Here's the drawing with two shaded views (mm, measured from the low corner). I have some questions. A direction names the side the tool comes from. Give positions to 0.01 mm unless a question says otherwise; leave off trailing zeros. Loops run counter-clockwise (first coordinate to the right, second up) from the corner with the lowest first, then second, coordinate; pieces in that order, holes last.
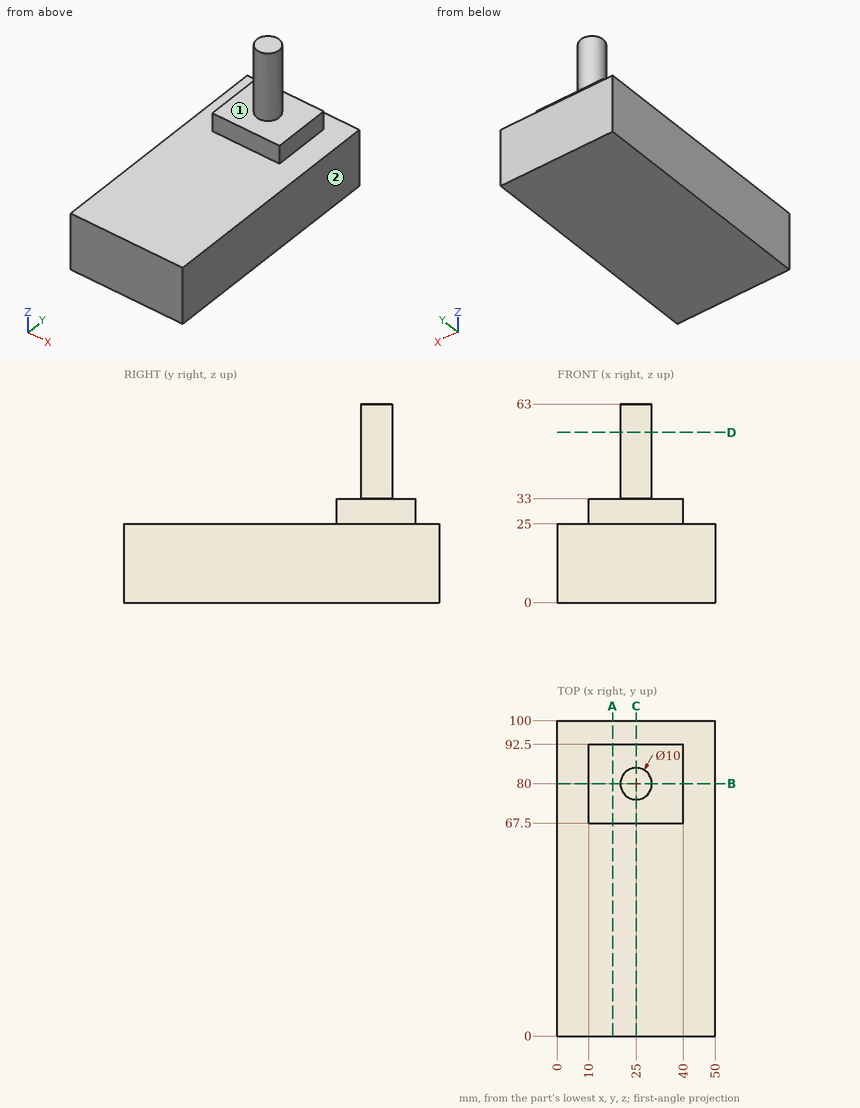
(1) Suppose I cut it at C-C on x = 25. List the corners of the cut face in (y, z) for me.
Returned:
outline: (0, 0) - (100, 0) - (100, 25) - (92.5, 25) - (92.5, 33) - (85, 33) - (85, 63) - (75, 63) - (75, 33) - (67.5, 33) - (67.5, 25) - (0, 25) - close
(2) Which directions (+Z, -Z, +X, -X, +Y, -Y) give clear straight access to the entire face, cutting with the end or side of a thin tool? Please do the marked faces 1 and 2.
Returned:
face 1: +Z
face 2: +Z, -Z, +X, +Y, -Y
(3) Please list where these lines run through material, in increasing order: probe 1 along Z at (x, y) = (18, 58); probe 2 along Y at (x, z) = (19, 29.5); probe 3 along Z at (x, y) = (32, 75.5).
Returned:
probe 1: z = 0 to 25
probe 2: y = 67.5 to 92.5
probe 3: z = 0 to 33
(4) Suppose I cut it at D-D on z = 54. List the corners of the cut face in (x, y) for me.
Returned:
outline: circle Ø10 at (25, 80)
(5) Suppose I cut it at B-B on y = 80. List the corners of the cut face in (x, z) for me.
Returned:
outline: (0, 0) - (50, 0) - (50, 25) - (40, 25) - (40, 33) - (30, 33) - (30, 63) - (20, 63) - (20, 33) - (10, 33) - (10, 25) - (0, 25) - close
(6) Suppose I cut it at A-A on x = 17.5. List the corners of the cut face in (y, z) for me, plus the area to 3 significant figures.
Returned:
outline: (0, 0) - (100, 0) - (100, 25) - (92.5, 25) - (92.5, 33) - (67.5, 33) - (67.5, 25) - (0, 25) - close
area: 2,700 mm2
(7) Will these pins go through, and if not, where does the flat tip stop? P1, Ø3, axis at x = 43.5, y = 43.5, coming from the +Z side; P2, Ø4, axis at y = 81, z = 29.5, coming from the -X side; P3, Ø2.5, axis at x = 29.5, z = 27.5, coming from the -Y side.
Returned:
P1: stops at z = 25
P2: stops at x = 10
P3: stops at y = 67.5
